Study the drawing (mm; zero at the part's minimum x, y, z) and answer. Coordinates: 2 decimals unless noted, no trailing zeros. Order: outer loops, then holes, each group sorted by start corner. A loop starts at its lowest first (then second) coordinate and runs counter-clockwise, first axis right, second up. Notation, with made-up numbers: M 49.5,57.5 L 94.5,57.5 A19 ccw 94.5,62.5 Z; hole C -13.5,15 d8. An arc over 180 degrees is marked long. Use a Markdown table: item, result. Add a question column.
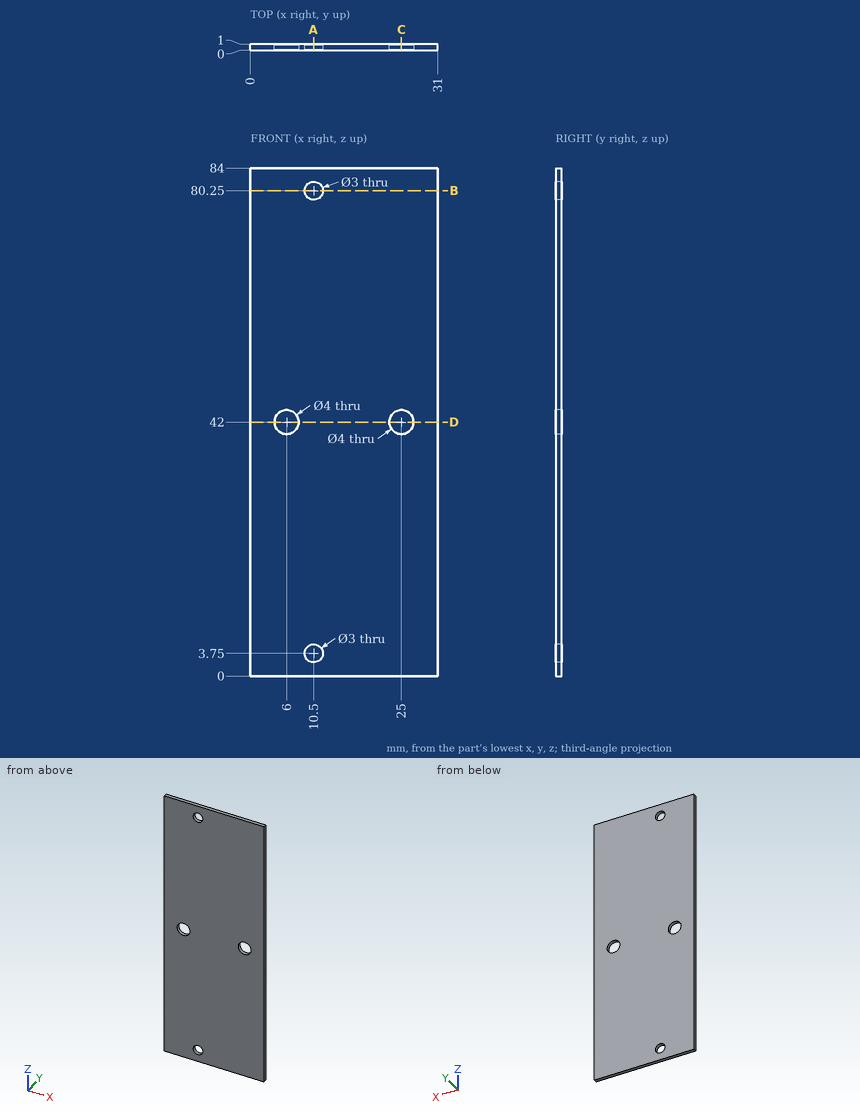
(1) Straight lines are drawn through the part: line 1 (Z direction, x = 10.5, y = 0.65); line 2 (Z direction, x = 25, y = 0.7); line 3 (X direction, y = 0.1, z = 41.5). For each, find the intervals that lie inside material, in ascending order.
(2) A cutting plane is placed at D-D on z = 42. Write down the section's boundary in (x, y).
(3) A cutting plane is placed at A-A on x = 10.5. Write down the section's boundary in (y, z), plus the area to 3 significant figures.
(4) A cutting plane is placed at C-C on x = 25. Write down the section's boundary in (y, z).
(5) A cutting plane is placed at B-B on z = 80.25. Write down the section's boundary in (x, y), plus the area to 3 significant figures.
From the geometry:
| question | item | result |
|---|---|---|
| 1 | line 1 | z = 0 to 2.25, 5.25 to 78.75, 81.75 to 84 |
| 1 | line 2 | z = 0 to 40, 44 to 84 |
| 1 | line 3 | x = 0 to 4.06, 7.94 to 23.06, 26.94 to 31 |
| 2 | outline | M 0,0 L 4,0 L 4,1 L 0,1 Z; M 8,0 L 23,0 L 23,1 L 8,1 Z; M 27,0 L 31,0 L 31,1 L 27,1 Z |
| 3 | outline | M 0,0 L 1,0 L 1,2.25 L 0,2.25 Z; M 0,5.25 L 1,5.25 L 1,78.75 L 0,78.75 Z; M 0,81.75 L 1,81.75 L 1,84 L 0,84 Z |
| 3 | area | 78.0 mm2 |
| 4 | outline | M 0,0 L 1,0 L 1,40 L 0,40 Z; M 0,44 L 1,44 L 1,84 L 0,84 Z |
| 5 | outline | M 0,0 L 9,0 L 9,1 L 0,1 Z; M 12,0 L 31,0 L 31,1 L 12,1 Z |
| 5 | area | 28.0 mm2 |
